Geometry check sheet. Reference: the model listing, model coordinates, mm. Face numbers are marked on the shaded views. Round coordinates to 2 decimals unless told otherwise and drop trailing zeros. Write each loop counter-clockwise with the first axis right and the second up, starting at its lowest first coordinate (ties: lowest second). Pieces come first, ordered by that corner, then holes.
Item 1: Draft check along X on the marked faces 1, 2 and 3. Enter one of: pulls with the +X half, pulls with the -X half, needs draft (parallel to the pull), parting line crosses it, or undercut.
Item 2: Depth check by flat-ended pin: P1, Ø2, axis at y = -35.5, z = -7, coming from the -X side; P2, Ø15, axis at x = 68.5, z = -12.5, coming from the -Y side; P3, Ø1, axis at y = -32, z = -17.5, coming from the -X side. Enter the tip coordinate at first touch or a pass-through.
Item 3: Cross-section at A-A (x = 0). Enter the section's corners in (y, z) (3 decimals).
Item 4: Cross-section at D-D (x = 88.9). Enter the section's corners in (y, z) (3 decimals).
Item 5: Scan lines: probe 1 along Z at (x, y) = (0, -38.5) (3 decimals); probe 2 along Y at (x, z) = (76, -8.5); probe 3 along Z at (x, y) = (82.5, -16.5). Record each from-to range of solid material in increasing order.
Item 6: Cross-section at C-C (y = -39.5). Enter the section's corners in (x, z) (3 decimals).
Item 7: Cross-section at B-B (y = -11). Enter the section's corners in (x, z) (3 decimals).
from build123d import *

# Parameters (mm, degrees)
F0_R     = 9.525
F1_DEPTH = 25.4
F2_DEPTH = 50.8
F3_SIZE  = 1.27


with BuildPart() as f1:
    # F0 (on Front) → F1 (new body)
    with BuildSketch(Plane.XZ):
        with BuildLine():
            ThreePointArc((90.376378, -17.437612), (101.785779, -11.840891), (106.4, 0))
            ThreePointArc((106.4, 0), (101.785779, 11.840891), (90.376378, 17.437612))
            ThreePointArc((90.376378, 17.437612), (71.4, 0), (90.376378, -17.437612))
        make_face()
        with Locations((88.9, 0)):
            Circle(F0_R, mode=Mode.SUBTRACT)
        with BuildLine():
            ThreePointArc((90.376378, -17.437612), (71.4, 0), (90.376378, 17.437612))
            Line((90.376378, 17.437612), (2.109111, 24.910874))
            ThreePointArc((2.109111, 24.910874), (18.408256, 16.915558), (25, 0))
            ThreePointArc((25, 0), (18.408256, -16.915558), (2.109111, -24.910874))
            Line((2.109111, -24.910874), (90.376378, -17.437612))
        make_face()
        with BuildLine():
            ThreePointArc((25, 0), (18.408256, 16.915558), (2.109111, 24.910874))
            ThreePointArc((2.109111, 24.910874), (-25, 0), (2.109111, -24.910874))
            ThreePointArc((2.109111, -24.910874), (18.408256, -16.915558), (25, 0))
        make_face()
        Circle(F0_R, mode=Mode.SUBTRACT)
    extrude(amount=F1_DEPTH)

    # F0 (on Front) → F2 (join)
    with BuildSketch(Plane.XZ):
        with BuildLine():
            ThreePointArc((25, 0), (18.408256, 16.915558), (2.109111, 24.910874))
            ThreePointArc((2.109111, 24.910874), (-25, 0), (2.109111, -24.910874))
            ThreePointArc((2.109111, -24.910874), (18.408256, -16.915558), (25, 0))
        make_face()
        Circle(F0_R, mode=Mode.SUBTRACT)
    extrude(amount=F2_DEPTH)

    # F3
    f3_edges = [f1.edges().sort_by_distance(p)[0] for p in [
        (-9.525, -50.8, 0),
        (-2.109111, -50.8, 24.910874),
        (79.375, -25.4, 0),
    ]]
    chamfer(f3_edges, length=F3_SIZE)


solid = f1.part
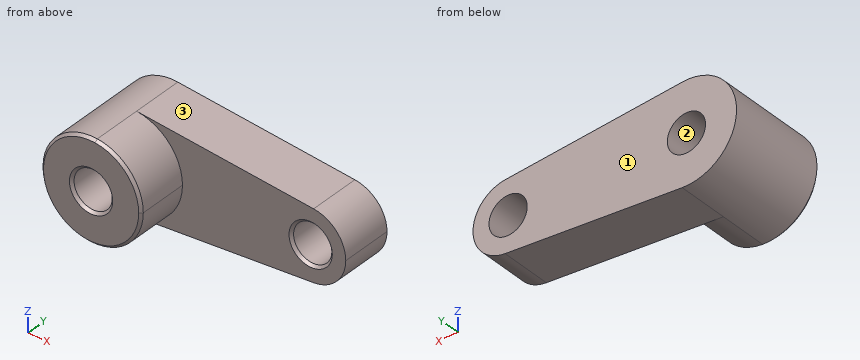
Resolved:
1. face 1: needs draft
1. face 2: undercut
1. face 3: pulls with the +X half
2. P1: stops at x = -24.27
2. P2: stops at y = -25.4
2. P3: stops at x = -18.33
3. outline: (-50.8, -23.73) - (-49.53, -25) - (0, -25) - (0, -9.525) - (-49.53, -9.525) - (-50.8, -10.795) - close; (-50.8, 10.795) - (-49.53, 9.525) - (0, 9.525) - (0, 25) - (-49.53, 25) - (-50.8, 23.73) - close
4. outline: (-25.4, -17.563) - (0, -17.563) - (0, -9.525) - (-24.13, -9.525) - (-25.4, -10.795) - close; (-25.4, 10.795) - (-24.13, 9.525) - (0, 9.525) - (0, 17.563) - (-25.4, 17.563) - close
5. probe 1: z = -25 to -9.525, 9.525 to 25
5. probe 2: y = -25.4 to 0
5. probe 3: z = -18.1 to -7.05, 7.05 to 18.1
6. outline: circle Ø50 at (0, 0); hole circle Ø19.05 at (0, 0)
7. outline: (2.109, -24.911) - (90.376, -17.438) arc R17.5 ccw to (90.376, 17.438) - (2.109, 24.911) arc R25 ccw (long way) to start; hole circle Ø19.05 at (0, 0); hole circle Ø19.05 at (88.9, 0)
